Here's how the part is built. I have some questions about the finished solid (model axes, mm). Face numbers are marked on the shaded views. Round coordinates to 2 decimals unless told otherwise and drop trailing zeros. Loops run counter-clockwise (first coordinate to the right, second up) from the corner with the lowest first, then second, coordinate; pieces in that order, holes last. Notation, with made-up numbers: M -14,29 L 11,29 A25 ccw 11,62 Z; hole C -36.75,64.25 d7. An arc over 180 degrees is marked long. Answer as a JSON object with one key per item and string values.
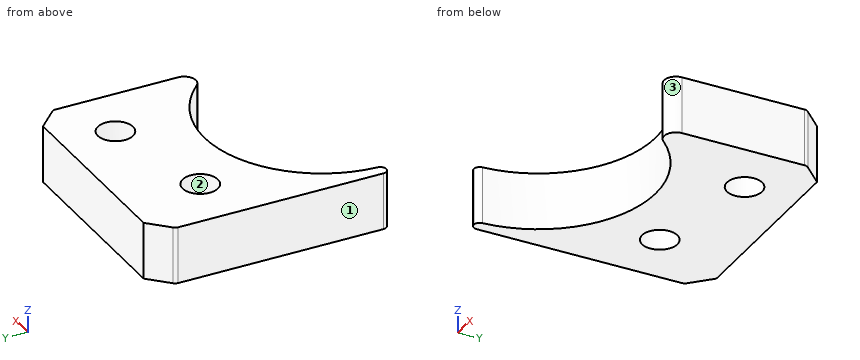
from build123d import *

# Parameters (mm, degrees)
BOSS_EXTRUDE1_DEPTH = 4.87
SKETCH2_R           = 1.5
CUT_EXTRUDE1_DEPTH  = 4.87
CHAMFER1_SIZE       = 1.8
FILLET1_R           = 0.5
FILLET2_R           = 1


with BuildPart() as part:
    # Sketch1 → Boss-Extrude1 (new body)
    with BuildSketch(Plane.XY):
        with BuildLine():
            Line((0, 0), (1, 0))
            ThreePointArc((1, 0), (8.763932023, 9.746794345), (20, 4.358898944))
            Line((20, 4.358898944), (20, 20))
            Line((20, 20), (0, 20))
            Line((0, 20), (0, 0))
        make_face()
    extrude(amount=BOSS_EXTRUDE1_DEPTH)

    # Sketch2 → Cut-Extrude1 (cut)
    with BuildSketch(Plane.XY.offset(4.87)):
        with Locations((5, 13.5)):
            Circle(SKETCH2_R)
        with Locations((15, 15.5)):
            Circle(SKETCH2_R)
    extrude(amount=-CUT_EXTRUDE1_DEPTH, mode=Mode.SUBTRACT)

    # Chamfer1
    chamfer1_edges = [part.edges().sort_by_distance(p)[0] for p in [
        (0, 20, 2.435),
        (20, 20, 2.435),
    ]]
    chamfer(chamfer1_edges, length=CHAMFER1_SIZE)

    # Fillet1
    fillet1_edges = [part.edges().sort_by_distance(p)[0] for p in [
        (0, 18.2, 2.435),
        (20, 18.2, 2.435),
        (1, 0, 2.435),
        (0, 0, 2.435),
    ]]
    fillet(fillet1_edges, radius=FILLET1_R)

    # Fillet2
    fillet2_edges = [part.edges().sort_by_distance(p)[0] for p in [
        (20, 4.358898944, 2.435),
    ]]
    fillet(fillet2_edges, radius=FILLET2_R)


solid = part.part
Item 1: I want a section at C-C on z = 3.85. Count the separate pieces of the cut face and the enclosed holes in it, plus the area to 3 significant figures.
Solution:
{"separate pieces": "1", "enclosed holes": "2", "area": "227 mm2"}
Item 2: I want a section at B-B on x = 5.5. List the corners of the cut face in (y, z) for me, plus the area to 3 significant figures.
Solution:
{"outline": "M 8.35,0 L 12.09,0 L 12.09,4.87 L 8.35,4.87 Z; M 14.91,0 L 20,0 L 20,4.87 L 14.91,4.87 Z", "area": "43.0 mm2"}
Item 3: If I drill on L1, parallel to X at y = 8.5, z = 2.1; L2, parallel to Y at x = 5, z = 3.1; L3, parallel to Y at x = 15, z = 2.35, over which ranges is the centre line in solid material (lowest first)? Write a range as from..to.
Solution:
{"L1": "x = 0..5.73, 16.27..20", "L2": "y = 8..12, 15..20", "L3": "y = 9.17..14, 17..20"}
Item 4: We'd pull the mould along Y, two halves only. Please class the marked faces 1, 2 and 3: +Y half, -Y half, draft (parallel to the pull), parting line (faces both ways), or undercut.
Solution:
{"face 1": "draft", "face 2": "undercut", "face 3": "-Y half"}
Item 5: I want a section at D-D on x = 12.75. List the corners of the cut face in (y, z) for me.
Solution:
{"outline": "M 9.85,0 L 20,0 L 20,4.87 L 9.85,4.87 Z"}
Item 6: I want a section at A-A on y = 13.5. List the corners of the cut face in (x, z) for me, plus the area to 3 significant figures.
Solution:
{"outline": "M 0,0 L 3.5,0 L 3.5,4.87 L 0,4.87 Z; M 6.5,0 L 20,0 L 20,4.87 L 6.5,4.87 Z", "area": "82.8 mm2"}
Item 7: For P1, Ø1.5, axis at x = 6, z = 4, coming from the -Y side; P2, Ø1.5, axis at x = 14.5, z = 1.5, coming from the -Y side, each with a flat end and sliding along its axis, tell me the tip position at first contact or that it passes through.
Solution:
{"P1": "stops at y = 8.18", "P2": "stops at y = 9.05"}
